Verification items for the finished model (mm, model axes). A direction names the side the tool comes from. Round coordinates to 2 decimals unless told otherwise and drop trailing zeros. Loops run counter-clockwise (first coordinate to the right, second up) from the corner with the lowest first, then second, coordinate; pieces in that order, holes last. Notation, with made-up numbers: (70.5, -2.5) -> (113.5, -2.5) arc R6 ccw to (113.5, 6.5) -> close; hole circle Ø2 at (-9.75, 81). An arc over 180 degrees is marked (long way). Use CSV: the item, a comma, the result in double quotes. Start each with the question number.
```python
from build123d import *

# Parameters (mm, degrees)
F0_R     = 10.5
F1_DEPTH = 5
F2_R     = 5.75
F3_DEPTH = 0.5
F4_R     = 4
F5_DEPTH = 3.5


with BuildPart() as f1:
    # F0 (on Top) → F1 (new body)
    with BuildSketch(Plane.XY):
        Circle(F0_R)
    extrude(amount=F1_DEPTH)

    # F2 (on face) → F3 (join)
    with BuildSketch(Plane.XY.offset(5)):
        Circle(F2_R)
    extrude(amount=F3_DEPTH)

    # F4 (on face) → F5 (cut)
    with BuildSketch(Plane.XY.offset(5.5)):
        Circle(F4_R)
    extrude(amount=-F5_DEPTH, mode=Mode.SUBTRACT)

    # F6 (on Front) → F7 (revolve, cut)
    with BuildSketch(Plane.XZ):
        with BuildLine():
            Line((0, 1), (0, -39))
            ThreePointArc((0, -39), (20, -19), (0, 1))
        make_face()
    revolve(axis=Axis((0, 0, -19), (0, 0, -1)), mode=Mode.SUBTRACT)


solid = f1.part
```
Q1. Tool access check on faces 1 (the face through (-0.867, -3.905, 3.774)), 2 (the face through (2, -4, 5.5)). Record the directions out of +Z, -Z, +X, -X, +Y, -Y that give a thin tool (end or side, any length) a straight path to the whole face; none if there is none.
Q2. Cross-section at A-A (x = 0). Record the boundary of the cut face in (y, z) (3 decimals), and give its area (3 significant figures).
Q3. Thickness scan on L1, parallel to Y at x = 0, z = 4.55; L2, parallel to Z at x = -4, y = 6.75; L3, parallel to X at y = 0.5, z = 2.8. Record the ranges inside material, lowest first. Write a range as from..to.
Q4. Cross-section at C-C (z = 4). Record the boundary of the cut face in (x, y), and give its area (3 significant figures).
Q5. Cross-section at D-D (x = -4.25). Record the boundary of the cut face in (y, z), and give its area (3 significant figures).
Q6. Depth check by flat-ended pin: pin 1 Ø7 at (x, y) = (0, 0) entering from -Z; pin 2 Ø4 at (x, y) = (7.5, 1) entering from -Z; pin 3 Ø2 at (x, z) = (-3, 2) entering from -Y. Enter the tip coordinate at first touch or a pass-through.
Answer list:
1,face 1,"+Z"
1,face 2,"+Z, +X, -X, +Y, -Y"
2,outline,"(-10.5, 0) -> (-6.245, 0) arc R20 cw to (6.245, 0) -> (10.5, 0) -> (10.5, 5) -> (5.75, 5) -> (5.75, 5.5) -> (4, 5.5) -> (4, 2) -> (-4, 2) -> (-4, 5.5) -> (-5.75, 5.5) -> (-5.75, 5) -> (-10.5, 5) -> close"
2,area,"74.4 mm2"
3,L1,"y = -10.5..-4, 4..10.5"
3,L2,"z = 0..5"
3,L3,"x = -10.49..-3.97, 3.97..10.49"
4,outline,"circle Ø21 at (0, 0); hole circle Ø8 at (0, 0)"
4,area,"296 mm2"
5,outline,"(-9.6, 0) -> (-4.58, 0) arc R19.54 cw to (4.58, 0) -> (9.6, 0) -> (9.6, 5) -> (3.87, 5) -> (3.87, 5.5) -> (-3.87, 5.5) -> (-3.87, 5) -> (-9.6, 5) -> close"
5,area,"96.6 mm2"
6,pin 1,"stops at z = 0.69"
6,pin 2,"stops at z = 0"
6,pin 3,"stops at y = -10.31"
